Source: CAD feature listing. Evaluate the final solid. Frame: model axes, mm. Face numbers are marked on the shaded views. A direction names the side the tool comes from. Coordinates: 2 decimals unless noted, no trailing zeros. Write each loop counter-clockwise with the first axis right and the second up, starting at its lowest first coordinate (ties: lowest second). Pieces come first, ordered by that corner, then holes. Notation, with made-up numbers: (15.25, 10) - (69.25, 10) arc R25 ccw to (69.25, 33) - close; hole circle Ø7 at (-36, -31). An arc over 180 degrees is marked (long way). One line per question, with ' | ' between items.
from build123d import *

# Parameters (mm, degrees)
F0_R      = 5.55625
F0_R_2    = 3.96875
F1_DEPTH  = 5.55625
F3_DEPTH  = 5.55625
F4_DEPTH  = 5.55625
F2_W      = 20.6375
F2_H      = 3.175
F2_W_2    = 20.66925
F5_DEPTH  = 0.396875
F6_DEPTH  = 0.396875
F7_DEPTH  = 0.396875
F8_DEPTH  = 0.396875
F9_DEPTH  = 0.0141922326
F10_DEPTH = 0.0141922326


with BuildPart() as f1:
    # F0 (on Front) → F1 (new body)
    with BuildSketch(Plane.XZ):
        Circle(F0_R)
        Circle(F0_R_2, mode=Mode.SUBTRACT)
    extrude(amount=F1_DEPTH)

    # F0 (on Front) → F3 (join)
    with BuildSketch(Plane.XZ):
        Circle(F0_R)
        Circle(F0_R_2, mode=Mode.SUBTRACT)
    extrude(amount=F3_DEPTH)

    # F4 (add): a face of the model
    f4_faces = [f1.faces().sort_by_distance(p)[0] for p in [
        (-5.3990955179, 0, 0),
    ]]
    extrude(f4_faces, amount=F4_DEPTH)

    # F2 (on Top) → F5 (join)
    with BuildSketch(Plane.XY):
        with Locations((15.875, 0)):
            Rectangle(F2_W, F2_H)
        with Locations((-15.890875, 0)):
            Rectangle(F2_W_2, F2_H)
    extrude(amount=F5_DEPTH)

    # F6 (add): a face of the model
    f6_faces = [f1.faces().sort_by_distance(p)[0] for p in [
        (15.875, 0, 0),
    ]]
    extrude(f6_faces, amount=F6_DEPTH)

    # F2 (on Top) → F7 (join)
    with BuildSketch(Plane.XY):
        with Locations((-15.890875, 0)):
            Rectangle(F2_W_2, F2_H)
    extrude(amount=F7_DEPTH)

    # F8 (add): a face of the model
    f8_faces = [f1.faces().sort_by_distance(p)[0] for p in [
        (-15.890875, 0, 0),
    ]]
    extrude(f8_faces, amount=F8_DEPTH)

    # F9 (add, through all): faces of the model
    f9_faces = [f1.faces().sort_by_distance(p)[0] for p in [
        (5.55625, 0, 0.1984375),
        (5.55625, 0, -0.1984375),
    ]]
    extrude(f9_faces, amount=F9_DEPTH)

    # F10 (add, through all): faces of the model
    f10_faces = [f1.faces().sort_by_distance(p)[0] for p in [
        (-5.55625, 0, 0.1984375),
        (-5.55625, 0, -0.1984375),
    ]]
    extrude(f10_faces, amount=F10_DEPTH)

    # F11: union 


solid = f1.part
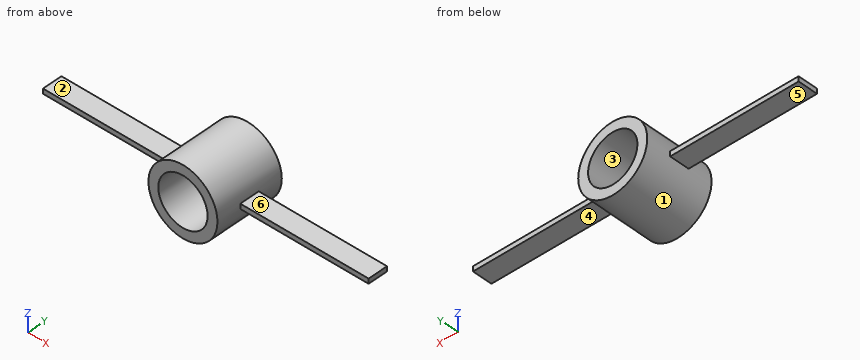
Item 1: Mould query, pull axis X, two halves, no side actions, for the marked faces 1, 2 and 3. Classes: pulls with the +X half, pulls with the -X half, needs draft (parallel to the pull), parting line crosses it, or undercut.
Check sheet entries:
face 1: parting line crosses it | face 2: needs draft | face 3: undercut
Item 2: Cut plane B-B on x = 0. Return loops of the section in (y, z).
Check sheet entries:
outline: (-5.56, -5.56) - (5.56, -5.56) - (5.56, -3.97) - (-5.56, -3.97) - close; (-5.56, 3.97) - (5.56, 3.97) - (5.56, 5.56) - (-5.56, 5.56) - close
Item 3: Access query for the marked faces 4, 5 and 6. Directions: +Z, -Z, +X, -X, +Y, -Y. A direction counts if a zero-diameter tool reaches every point of the face in a straight line with its end or side. Return the directions, or none.
Check sheet entries:
face 4: -Z, +X, +Y, -Y | face 5: -Z, -X, +Y, -Y | face 6: +Z, +X, +Y, -Y
Item 4: Cut plane A-A on y = 0.25. Return loops of the section in (x, z).
Check sheet entries:
outline: (-26.23, -0.4) - (-5.54, -0.4) arc R5.56 ccw to (5.54, -0.4) - (26.19, -0.4) - (26.19, 0.4) - (5.54, 0.4) arc R5.56 ccw to (-5.54, 0.4) - (-26.23, 0.4) - close; hole circle Ø7.94 at (0, 0)
Item 5: Cut plane C-C on z = -1. Return loops of the section in (x, y), and give its area (3 significant figures).
Check sheet entries:
outline: (-5.47, -5.56) - (-3.84, -5.56) - (-3.84, 5.56) - (-5.47, 5.56) - close; (3.84, -5.56) - (5.47, -5.56) - (5.47, 5.56) - (3.84, 5.56) - close | area: 36.1 mm²
Item 6: Ray query, line 1 along Z through (x, y) = (0, 0.75); line 2 along X through (y, z) = (-2.25, -1.5); line 3 along Z through (x, y) = (-16, -0.75). Return the intervals inside material, ascending. Write a range as [from, to].
Check sheet entries:
line 1: [-5.56, -3.97], [3.97, 5.56] | line 2: [-5.35, -3.67], [3.67, 5.35] | line 3: [-0.4, 0.4]
Item 7: Pin query (flat end, axial travel): pin 1 Ø1.6 at (x, y) = (-13, 0) entering from -Z; pin 2 Ø2 at (x, y) = (20, -1.5) entering from +Z; pin 3 Ø3 at (x, z) = (-17, 0.5) entering from -Y; pin 4 Ø3 at (x, z) = (19, 2.5) entering from -Y. Return the tip coordinate at first contact, or that it passes through.
Check sheet entries:
pin 1: z = -0.4 | pin 2: z = 0.4 | pin 3: y = -1.59 | pin 4: through
Item 8: Cut plane D-D on x = -13. Return loops of the section in (y, z), and give its area (3 significant figures).
Check sheet entries:
outline: (-1.59, -0.4) - (1.59, -0.4) - (1.59, 0.4) - (-1.59, 0.4) - close | area: 2.52 mm²
